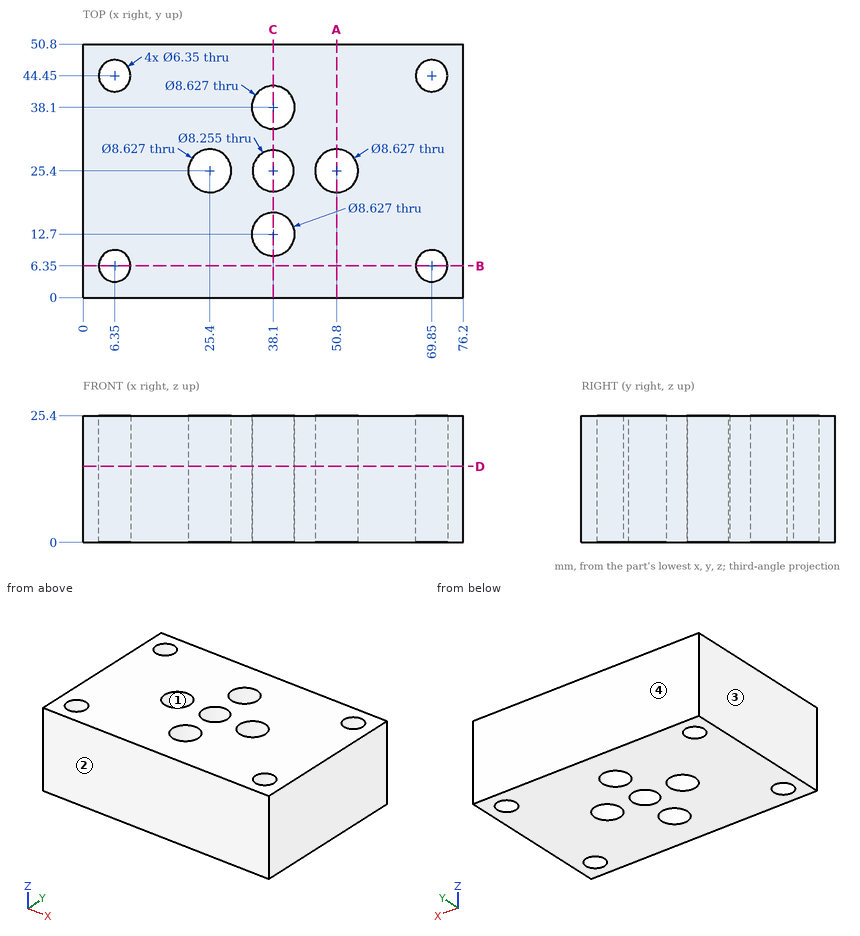
Input: dimensioned drawing with shaded views. Units: mm. Origin: part minimum x, y, z. Give positions to 0.01 mm unless a question says otherwise; leave off trailing zeros. Write each loop counter-clockwise with the first axis right and the second up, starting at its lowest first coordinate (ties: lowest second). Pieces come first, ordered by that corner, then holes. Notation, with made-up numbers: M 22,30.25 L 35,30.25 A26 ccw 35,51.25 Z; hole C 88.25,54.25 d4. An arc over 180 degrees is marked long. Write item = value, one per line. Start each with the question number.
1) Material intervals for line 1 along Y through (x, z) = (38.1, 11); line 2 along Y through (x, z) = (69.85, 18) (1 decimal); line 3 along Y through (x, z) = (50.8, 16.5), sorted ascending. Write a range as [from, to].
2) Draft query along Y for the marked faces 1, 2, 3 and 4. Return one class per face: +Y half, -Y half, draft (parallel to the pull), parting line (faces both ways), or undercut.
3) Cut plane A-A on x = 50.8. Return the cut outline in (y, z).
4) Cut plane B-B on y = 6.35. Return the cut outline in (x, z) (1 decimal), then the cut area to 3 significant figures.
5) First-contact query: pin 1 Ø5.5 at (x, y) = (6.35, 6.35) entering from -Z. Flat tip, straight axial feed; report the tip coordinate or a pass-through.
6) Cut plane D-D on z = 15.25. Count the separate pieces of the cut face and the enclosed holes in it, then the cut area to 3 significant figures.
7) Cut plane C-C on x = 38.1. Return the cut outline in (y, z).
Solved:
q1.line_1 = [0, 8.39], [17.01, 21.27], [29.53, 33.79], [42.41, 50.8]
q1.line_2 = [0, 3.2], [9.5, 41.3], [47.6, 50.8]
q1.line_3 = [0, 21.09], [29.71, 50.8]
q2.face_1 = undercut
q2.face_2 = -Y half
q2.face_3 = draft
q2.face_4 = +Y half
q3.outline = M 0,0 L 21.09,0 L 21.09,25.4 L 0,25.4 Z; M 29.71,0 L 50.8,0 L 50.8,25.4 L 29.71,25.4 Z
q4.outline = M 0,0 L 3.2,0 L 3.2,25.4 L 0,25.4 Z; M 9.5,0 L 66.7,0 L 66.7,25.4 L 9.5,25.4 Z; M 73,0 L 76.2,0 L 76.2,25.4 L 73,25.4 Z
q4.area = 1,610 mm2
q5.pin_1 = through
q6.separate_pieces = 1
q6.enclosed_holes = 9
q6.area = 3,460 mm2
q7.outline = M 0,0 L 8.39,0 L 8.39,25.4 L 0,25.4 Z; M 17.01,0 L 21.27,0 L 21.27,25.4 L 17.01,25.4 Z; M 29.53,0 L 33.79,0 L 33.79,25.4 L 29.53,25.4 Z; M 42.41,0 L 50.8,0 L 50.8,25.4 L 42.41,25.4 Z
